Input: part model. Units: mm. Frame: model coordinates. Face numbers are marked on the shaded views. A direction names the side the tool comes from. Round coordinates to 2 decimals unless told otherwise and drop trailing zeros. Write each loop counter-clockwise with the first axis right and the second up, starting at its lowest first coordinate (ties: lowest second). Pieces come first, ordered by that corner, then holes. Notation, with made-up numbers: (84, -23.75) - (109, -23.75) arc R13 cw to (109, -19.75) - close; hole circle Ø10 at (73, -15). An arc over 180 degrees is marked (long way). Use one line per item in the form item = value.
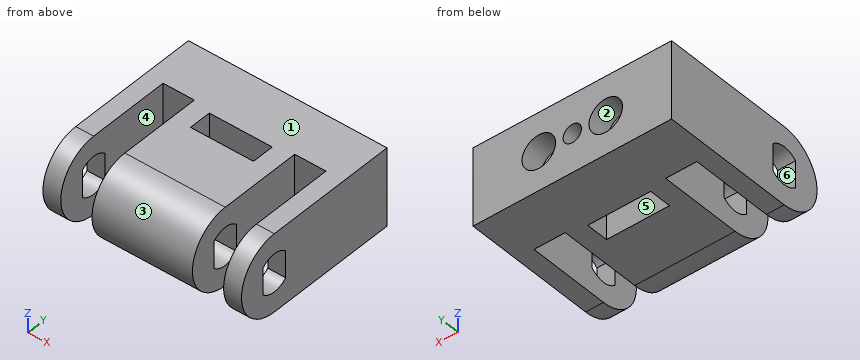
Autodesk Inventor part; units mm, degrees
ref_plane "РабПлоскость1" through (22.5, 0, 17.5) normal (1, 0, 0) x (0, 0, -1)
ref_plane "YZ Plane" through (0, 0, 0) normal (1, 0, 0) x (0, 1, 0)
ref_plane "XZ Plane" through (0, 0, 0) normal (0, 1, 0) x (-1, 0, 0)
sketch "Эскиз1" plane through (0, 0, 0) normal (1, 0, 0) x (0, 1, 0)
  line L0 (-6, -6.0208) -> (-6, 6.0208)
  arc A0 (-6, -6.0208) -> (6, -6.0208) centre (0, 0) ccw
  line L1 (6, 6.0208) -> (6, -6.0208)
  arc A1 (6, 6.0208) -> (-6, 6.0208) centre (0, 0) ccw
  circle A2 centre (0, 0) radius 17.5
  line L2 (0, 17.5) -> (60, 17.5)
  line L3 (60, 17.5) -> (60, -17.5)
  line L4 (60, -17.5) -> (0, -17.5)
  line L5 (0, -17.5) -> (0, -8.5)
  line L6 (0, 8.5) -> (0, 17.5)
  dimension "d0" = 35
  dimension "d1" = 60
extrude "Выдавливание1" add sketch "Эскиз1" along normal blind 45 contours A0 L5 A2 L6 A1 L0 | A0 L1 A1 L6 A2 L5 | A2 L2 L3 L4
sketch "Эскиз2" plane through (45, 0, 0) normal (1, 0, 0) x (0, 0, -1)
  line L0 (17.5, 60) -> (-17.5, 60)
  line L1 (17.5, 0) -> (17.5, 60)
  line L2 (-17.5, 60) -> (17.5, 60)
  line L3 (17.5, 60) -> (17.5, 37)
  line L4 (17.5, 37) -> (-17.5, 37)
  line L5 (-17.5, 37) -> (-17.5, 60)
  point P0 (0, 0)
  dimension "d4" = 23
extrude "Выдавливание2" add sketch "Эскиз2" along normal blind 22
ref_plane "РабПлоскость1" through (22.5, 0, 17.5) normal (1, 0, 0) x (0, 0, -1)
mirror "Зеркальное отражение1" about plane through (22.5, 0, 17.5) normal (1, 0, 0) of "Выдавливание2"
sketch "Эскиз3" plane through (45, 0, 0) normal (1, 0, 0) x (0, 0, -1)
  arc A0 (6.0208, -6) -> (6.0208, 6) centre (0, 0) ccw
  line L0 (6.0208, -6) -> (-6.0208, -6)
  arc A1 (-6.0208, 6) -> (-6.0208, -6) centre (0, 0) ccw
  line L1 (6.0208, 6) -> (-6.0208, 6)
  line L2 (17.5, 37) -> (-17.5, 37)
  line L3 (-17.5, 37) -> (-17.5, 0)
  arc A2 (-17.5, 0) -> (17.5, 0) centre (0, 0) ccw
  line L4 (17.5, 0) -> (17.5, 37)
sketch "Эскиз4" plane through (67, 0, 0) normal (1, 0, 0) x (0, 0, -1)
  arc A0 (6.0208, -6) -> (6.0208, 6) centre (0, 0) ccw
  line L0 (6.0208, -6) -> (-6.0208, -6)
  arc A1 (-6.0208, 6) -> (-6.0208, -6) centre (0, 0) ccw
  line L1 (6.0208, 6) -> (-6.0208, 6)
  line L2 (17.5, 37) -> (-17.5, 37)
  line L3 (-17.5, 37) -> (-17.5, 0)
  arc A2 (-17.5, 0) -> (17.5, 0) centre (0, 0) ccw
  line L4 (17.5, 0) -> (17.5, 37)
extrude "Выдавливание3" add sketch "Эскиз4" against normal blind 8
mirror "Зеркальное отражение2" about plane through (22.5, 0, 17.5) normal (1, 0, 0) of "Выдавливание3"
sketch "Эскиз5" plane through (67, 60, 17.5) normal (0, 1, 0) x (1, 0, 0)
  line L0 (-89, 35) -> (-89, 0)
  line L1 (-89, 35.1034) -> (-89, 0)
  line L2 (-89, 0) -> (-89, 35.1034)
  line L3 (-89, 35) -> (0, 35)
  line L4 (-89, 35) -> (0, 35)
  line L5 (-89, 17.5517) -> (-44.5, 17.5517)
  circle A0 centre (-44.5, 17.5517) radius 4.1
  line L6 (-44.5, 17.5517) -> (-59.5, 17.5517)
  circle A1 centre (-59.5, 17.5517) radius 7.5
  line L7 (-44.5, 17.5517) -> (-29.5, 17.5517)
  circle A2 centre (-29.5, 17.5517) radius 7.5
  point P0 (-67, 17.5)
  dimension "d9" = 8.2
  dimension "d10" = 15
  dimension "d11" = 15
  dimension "d12" = 15
  dimension "d13" = 15
extrude "Выдавливание4" cut sketch "Эскиз5" against normal blind 10 contours L5 A1 | L5 A1 | A2
sketch "Эскиз6" plane through (67, 60, 17.5) normal (0, 1, 0) x (1, 0, 0)
  line L0 (-89, 35) -> (-89, 0)
  line L1 (-89, 35.1034) -> (-89, 0)
  line L2 (-89, 0) -> (-89, 35.1034)
  line L3 (-89, 35) -> (0, 35)
  line L4 (-89, 35) -> (0, 35)
  line L5 (-89, 17.5517) -> (-44.5, 17.5517)
  circle A0 centre (-44.5, 17.5517) radius 4.1
  line L6 (-44.5, 17.5517) -> (-59.5, 17.5517)
  circle A1 centre (-59.5, 17.5517) radius 7.5
  line L7 (-44.5, 17.5517) -> (-29.5, 17.5517)
  circle A2 centre (-29.5, 17.5517) radius 7.5
  point P0 (-67, 17.5)
  point P1 (-67, 17.5)
  dimension "d16" = 8.2
  dimension "d17" = 15
  dimension "d18" = 15
  dimension "d19" = 15
  dimension "d20" = 15
extrude "Выдавливание5" cut sketch "Эскиз6" against normal blind 35 contours A0 L7 L5 | L5 L7 A0
sketch "Эскиз7" plane through (0, 0, 17.5) normal (0, 0, 1) x (1, 0, 0)
  line L0 (18.4, 60) -> (18.4, 25)
  line L1 (26.6, 60) -> (26.6, 25)
  line L2 (0, 37) -> (0, 0)
  line L3 (45, 0) -> (0, 0)
  line L4 (45, 37) -> (45, 0)
  line L5 (45, 37) -> (59, 37)
  line L6 (59, 0) -> (59, 37)
  line L7 (67, 0) -> (59, 0)
  line L8 (67, 60) -> (67, 0)
  line L9 (-22, 60) -> (67, 60)
  line L10 (-22, 60) -> (-22, 0)
  line L11 (-22, 0) -> (-14, 0)
  line L12 (-14, 0) -> (-14, 37)
  line L13 (0, 37) -> (-14, 37)
  line L14 (18.4, 25) -> (26.6, 25)
  line L15 (18.4, 25) -> (8.4, 25)
  line L16 (8.4, 25) -> (8.4, 35)
  line L17 (8.4, 35) -> (36.6, 35)
  line L18 (36.6, 35) -> (36.6, 25)
  line L19 (26.6, 25) -> (36.6, 25)
  line L20 (18.4, 25) -> (26.6, 25)
  dimension "d23" = 10
  dimension "d24" = 10
  dimension "d25" = 28.2
  dimension "d26" = 10
extrude "Выдавливание6" cut sketch "Эскиз7" against normal blind 84.5 contours L17 L1 L14 L0 | L0 L15 L16 L17 | L17 L18 L19 L1
properties part number "joint1_level" material "Пластик АБС"
(1) Material intervals for L1, parallel to X at y = 2, z = 9.5; L2, parallel to X at y = 29.5, z = -5; L3, parallel to Z at x = 7, y = 53, sorted ascending.
Derived:
L1 = -22 to -14, 0 to 45, 59 to 67
L2 = -22 to -14, 0 to 8.4, 36.6 to 45, 59 to 67
L3 = -17.5 to -7.54, 7.43 to 17.5
(2) Cut plane A-A on x = 22.5. Output: boundary loops of the cut face in (y, z).
Derived:
outline = (0, -17.5) - (25, -17.5) - (25, 17.5) - (0, 17.5) arc R17.5 ccw to start; (35, -17.5) - (60, -17.5) - (60, -4.15) - (35, -4.15) - close; (35, 4.05) - (60, 4.05) - (60, 17.5) - (35, 17.5) - close; hole (-6, -6.02) arc R8.5 ccw to (6, -6.02) - (6, 6.02) arc R8.5 ccw to (-6, 6.02) - close
(3) Access query for the marked faces 4, 5 and 6. Directions: +Z, -Z, +X, -X, +Y, -Y. A direction counts if a zero-diameter tool reaches every point of the face in a straight line with its end or side. Return the directions, or none.
Derived:
face_4 = +Z, -Z, -Y
face_5 = +Z, -Z
face_6 = +X, -X
(4) Draft query along Z for the marked faces 1, 2 and 3. Return one class per face: released by +Z, released by -Z, zero draft, split by the parting line, or undercut.
Derived:
face_1 = released by +Z
face_2 = undercut
face_3 = split by the parting line
(5) Cut plane B-B on y = 7. Output: boundary loops of the cut face in (x, z).
Derived:
outline = (-22, -17.5) - (-14, -17.5) - (-14, 17.5) - (-22, 17.5) - close; (0, -17.5) - (45, -17.5) - (45, 17.5) - (0, 17.5) - close; (59, -17.5) - (67, -17.5) - (67, 17.5) - (59, 17.5) - close
(6) Cut plane C-C on z = -10.5. Output: boundary loops of the cut face in (x, y).
Derived:
outline = (-22, -14) - (-14, -14) - (-14, 37) - (0, 37) - (0, -14) - (45, -14) - (45, 37) - (59, 37) - (59, -14) - (67, -14) - (67, 60) - (-22, 60) - close; hole (8.4, 25) - (36.6, 25) - (36.6, 35) - (8.4, 35) - close
(7) Cut plane D-D on x = 34. Output: boundary loops of the cut face in (y, z), then the cut area to 3 significant figures.
Derived:
outline = (0, -17.5) - (25, -17.5) - (25, 17.5) - (0, 17.5) arc R17.5 ccw to start; (35, -17.5) - (60, -17.5) - (60, -6.68) - (50, -6.68) - (50, 6.58) - (60, 6.58) - (60, 17.5) - (35, 17.5) - close; hole (-6, -6.02) arc R8.5 ccw to (6, -6.02) - (6, 6.02) arc R8.5 ccw to (-6, 6.02) - close
area = 1,910 mm^2
(8) First-contact query: pin 1 Ø1.5 at (x, z) = (49, -11.5) entering from -Y; pin 2 Ø7.5 at (x, z) = (37.5, 2) entering from +Y; pin 3 Ø10 at (x, z) = (15.5, -9) entering from -Y. Flat tips, straight axial feed; report the tip coordinate or a pass-through.
Derived:
pin_1 = 37
pin_2 = 50
pin_3 = -17.04
